from build123d import *

# Parameters (mm, degrees)
F0_R     = 10
F1_DEPTH = 25
F2_DEPTH = 50
F3_SIZE  = 2
F4_R     = 8.379522
F5_DEPTH = 34.1921


with BuildPart() as f1:
    # F0 (on Front) → F1 (new body)
    with BuildSketch(Plane.XZ):
        with BuildLine():
            ThreePointArc((2.083333, -24.913043), (18.399502, -16.92508), (25, 0))
            ThreePointArc((25, 0), (18.399502, 16.92508), (2.083333, 24.913043))
            ThreePointArc((2.083333, 24.913043), (-25, 0), (2.083333, -24.913043))
        make_face()
        Circle(F0_R, mode=Mode.SUBTRACT)
        with BuildLine():
            ThreePointArc((2.083333, 24.913043), (18.399502, 16.92508), (25, 0))
            ThreePointArc((25, 0), (18.399502, -16.92508), (2.083333, -24.913043))
            Line((2.083333, -24.913043), (91.458333, -17.43913))
            ThreePointArc((91.458333, -17.43913), (72.5, 0), (91.458333, 17.43913))
            Line((91.458333, 17.43913), (2.083333, 24.913043))
        make_face()
        with BuildLine():
            ThreePointArc((107.5, 0), (102.879651, 11.847556), (91.458333, 17.43913))
            ThreePointArc((91.458333, 17.43913), (72.5, 0), (91.458333, -17.43913))
            ThreePointArc((91.458333, -17.43913), (102.879651, -11.847556), (107.5, 0))
        make_face()
        with Locations((90, 0)):
            Circle(F0_R, mode=Mode.SUBTRACT)
    extrude(amount=F1_DEPTH)

    # F0 (on Front) → F2 (join)
    with BuildSketch(Plane.XZ):
        with BuildLine():
            ThreePointArc((2.083333, -24.913043), (18.399502, -16.92508), (25, 0))
            ThreePointArc((25, 0), (18.399502, 16.92508), (2.083333, 24.913043))
            ThreePointArc((2.083333, 24.913043), (-25, 0), (2.083333, -24.913043))
        make_face()
        Circle(F0_R, mode=Mode.SUBTRACT)
    extrude(amount=F2_DEPTH)

    # F3
    f3_edges = [f1.edges().sort_by_distance(p)[0] for p in [
        (-2.083333, -50, 24.913043),
        (-10, -50, 0),
        (80, -25, 0),
    ]]
    chamfer(f3_edges, length=F3_SIZE)

    # F4 (on Front) → F5 (cut)
    with BuildSketch(Plane.XZ):
        with Locations((56.286983, -8.367218)):
            Circle(F4_R)
    extrude(amount=F5_DEPTH, mode=Mode.SUBTRACT)


solid = f1.part
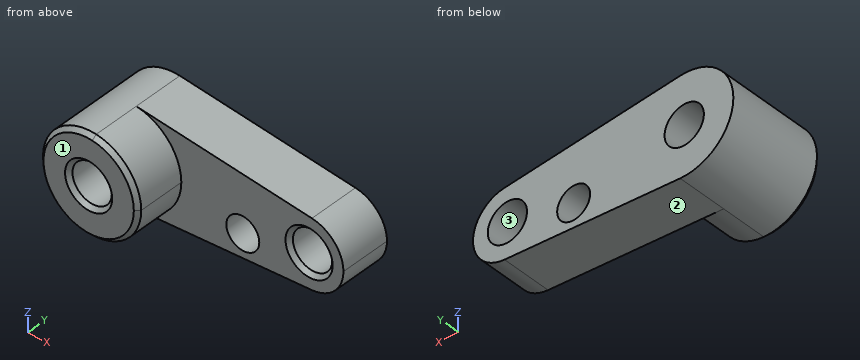
Input: part model. Units: mm. Frame: model coordinates. Face numbers are marked on the shaded views. Give positions to 0.01 mm unless a question says otherwise; leave off trailing zeros. Write each loop counter-clockwise with the first axis right and the second up, starting at its lowest first coordinate (ties: lowest second). Pieces come first, ordered by that corner, then holes.
Q1. Section D-D, the plane z = 3. State how many separate pieces and enclosed holes the cut face has, plus the area to 3 significant figures.
Q2. Pull-direction query (X, two-part tool) for the marked faces 1, 2 and 3; classes: pulls with the +X half, pulls with the -X half, needs draft (parallel to the pull), parting line crosses it, or undercut.
Q3. First-contact query: P1, Ø15, axis at x = 46, z = 10, coming from the -Y side; P2, Ø5, axis at x = -10, z = 4.5, coming from the -Y side; P3, Ø3, axis at y = -29, z = 20, coming from the -X side; P4, Ø5, axis at x = 22, y = -15, coming from the +Z side. Flat tips, straight axial feed; report the tip coordinate or a pass-through.
Q4. Section A-A, the plane x = 0. Output: boundary loops of the cut face in (y, z), plus the area to 3 significant figures.
Q5. Section C-C, the plane y = -34.5. Output: boundary loops of the cut face in (x, z), plus the area to 3 significant figures.
Q6. Section B-B, the plane y = -16. Output: boundary loops of the cut face in (x, z), plus the area to 3 significant figures.
Q7. Material intervals for probe 1 along X at (y, z) = (-20.5, 6); probe 2 along Y at (x, z) = (97, 11); probe 3 along Z at (x, y) = (52.5, -22), sorted ascending.
Filled in:
1. separate pieces: 3
1. enclosed holes: 0
1. area: 3,100 mm2
2. face 1: needs draft
2. face 2: pulls with the +X half
2. face 3: undercut
3. P1: stops at y = -25
3. P2: stops at y = -50
3. P3: stops at x = -16.82
3. P4: stops at z = 23.46
4. outline: (-50, -23) - (-48, -25) - (0, -25) - (0, -10) - (-48, -10) - (-50, -12) - close; (-50, 12) - (-48, 10) - (0, 10) - (0, 25) - (-48, 25) - (-50, 23) - close
4. area: 1,490 mm2
5. outline: (2.08, -24.91) arc R25 ccw to (25, 0) arc R25 ccw to (2.08, 24.91) arc R25 ccw (long way) to start; hole circle Ø20 at (0, 0)
5. area: 1,650 mm2
6. outline: (2.08, -24.91) - (91.46, -17.44) arc R17.5 ccw to (91.46, 17.44) - (2.08, 24.91) arc R25 ccw (long way) to start; hole circle Ø20 at (0, 0); hole circle Ø16.76 at (56.29, -8.37); hole circle Ø20 at (90, 0)
6. area: 4,450 mm2
7. probe 1: x = -24.27 to -8, 8 to 82, 98 to 106.44
7. probe 2: y = -25 to 0
7. probe 3: z = -20.7 to -15.84, -0.89 to 20.7
